```python
from build123d import *

# Parameters (mm, degrees)
SKETCH1_W               = 57.15
SKETCH1_H               = 18.542
BOSS_EXTRUDE1_DEPTH     = 19.05
CUT_EXTRUDE1_DEPTH      = 41.848617676
CUT_EXTRUDE1_DEPTH_BACK = 41.848617676
CUT_EXTRUDE2_DEPTH      = 4.572
CUT_EXTRUDE2_DEPTH_BACK = 4.572
CUT_EXTRUDE3_DEPTH      = 3.81
CUT_EXTRUDE3_DEPTH_BACK = 3.81
CUT_EXTRUDE5_DEPTH      = 44.89150133
FILLET1_R               = 3.175
SKETCH9_R               = 3.96875
CUT_EXTRUDE6_DEPTH      = 1.5875
SKETCH10_W              = 22.225
SKETCH10_H              = 6.096
CUT_EXTRUDE7_DEPTH      = 41.503184716
FILLET2_R               = 3.175
FILLET3_R               = 0.79375


with BuildPart() as part:
    # Sketch1 → Boss-Extrude1 (new body)
    with BuildSketch(Plane.XY):
        with Locations((6.35, 0)):
            Rectangle(SKETCH1_W, SKETCH1_H)
    extrude(amount=BOSS_EXTRUDE1_DEPTH)

    # Sketch3 → Cut-Extrude1 (cut, two sides: drawn at the far end of the back side and taken through both)
    with BuildSketch(Plane(origin=(0, 0, 0), x_dir=(1, 0, 0), z_dir=(0, 1, 0)).offset(-CUT_EXTRUDE1_DEPTH_BACK)):
        with BuildLine():
            Line((-5.1435, -19.05), (-5.1435, -14.2875))
            ThreePointArc((-5.1435, -14.2875), (0, -9.144), (5.1435, -14.2875))
            Line((5.1435, -14.2875), (5.1435, -19.05))
            ThreePointArc((5.1435, -19.05), (0, -24.1935), (-5.1435, -19.05))
        make_face()
    extrude(amount=CUT_EXTRUDE1_DEPTH + CUT_EXTRUDE1_DEPTH_BACK, mode=Mode.SUBTRACT)

    # Sketch5 → Cut-Extrude2 (cut, two sides: drawn at the far end of the back side and taken through both)
    with BuildSketch(Plane(origin=(0, 0, 0), x_dir=(1, 0, 0), z_dir=(0, 1, 0)).offset(-CUT_EXTRUDE2_DEPTH_BACK)):
        with BuildLine():
            Line((12.954, -14.2875), (12.954, -19.05))
            ThreePointArc((12.954, -19.05), (0, -32.004), (-12.954, -19.05))
            Line((-12.954, -19.05), (-12.954, -14.2875))
            ThreePointArc((-12.954, -14.2875), (0, -1.3335), (12.954, -14.2875))
        make_face()
        with BuildLine():
            Line((-6.731, -19.05), (-6.731, -14.2875))
            ThreePointArc((-6.731, -14.2875), (0, -7.5565), (6.731, -14.2875))
            Line((6.731, -14.2875), (6.731, -19.05))
            ThreePointArc((6.731, -19.05), (0, -25.781), (-6.731, -19.05))
        make_face(mode=Mode.SUBTRACT)
    extrude(amount=CUT_EXTRUDE2_DEPTH + CUT_EXTRUDE2_DEPTH_BACK, mode=Mode.SUBTRACT)

    # Sketch6 → Cut-Extrude3 (cut, two sides: drawn at the far end of the back side and taken through both)
    with BuildSketch(Plane(origin=(0, 0, 0), x_dir=(1, 0, 0), z_dir=(0, 1, 0)).offset(-CUT_EXTRUDE3_DEPTH_BACK)):
        with BuildLine():
            Line((-8.3185, -19.05), (-8.3185, -14.2875))
            ThreePointArc((-8.3185, -14.2875), (0, -5.969), (8.3185, -14.2875))
            Line((8.3185, -14.2875), (8.3185, -19.05))
            ThreePointArc((8.3185, -19.05), (0, -27.3685), (-8.3185, -19.05))
        make_face()
    extrude(amount=CUT_EXTRUDE3_DEPTH + CUT_EXTRUDE3_DEPTH_BACK, mode=Mode.SUBTRACT)

    # Sketch8 → Cut-Extrude5 (cut, through all)
    with BuildSketch(Plane.XZ.offset(9.271)):
        Polygon((-22.225, 19.05), (34.925, 19.05), (34.925, 6.803571429), align=None)
    extrude(amount=-CUT_EXTRUDE5_DEPTH, mode=Mode.SUBTRACT)

    # Fillet1
    fillet1_edges = [part.edges().sort_by_distance(p)[0] for p in [
        (-22.225, 0, 19.05),
        (34.925, 0, 6.803571429),
        (-22.225, 0, 0),
        (34.925, 0, 0),
    ]]
    fillet(fillet1_edges, radius=FILLET1_R)

    # Sketch9 → Cut-Extrude6 (cut)
    with BuildSketch(Plane(origin=(0, 0, 0), x_dir=(-1, 0, 0), z_dir=(0, 0, -1))):
        with Locations((-23.8125, 0)):
            Circle(SKETCH9_R)
    extrude(amount=-CUT_EXTRUDE6_DEPTH, mode=Mode.SUBTRACT)

    # Sketch10 → Cut-Extrude7 (cut, through all)
    with BuildSketch(Plane(origin=(0, 0, 0), x_dir=(-1, 0, 0), z_dir=(0, 0, -1))):
        with Locations((-23.8125, 6.223)):
            Rectangle(SKETCH10_W, SKETCH10_H)
        with Locations((-23.8125, -6.223)):
            Rectangle(SKETCH10_W, SKETCH10_H)
    extrude(amount=-CUT_EXTRUDE7_DEPTH, mode=Mode.SUBTRACT)

    # Fillet2
    fillet2_edges = [part.edges().sort_by_distance(p)[0] for p in [
        (12.7, 3.175, 5.783035714),
        (12.7, -3.175, 5.783035714),
    ]]
    fillet(fillet2_edges, radius=FILLET2_R)

    # Fillet3
    # the kernel refuses this fillet: 0.79375 mm, written as the material it adds along each edge
    with BuildSketch(Plane(origin=(-6.731, 4.572, 17.714232143), x_dir=(-1, 0, 0), z_dir=(0, 0, -1))) as fillet3_piece_1_section:
        with BuildLine():
            CenterArc((FILLET3_R, -FILLET3_R), FILLET3_R, 90, 90)
            Line((0, -FILLET3_R), (0, 0))
            Line((0, 0), (FILLET3_R, 0))
        make_face()
    fillet3_piece_1 = extrude(amount=3.426732143, mode=Mode.PRIVATE)
    fillet3_piece_1 = split(fillet3_piece_1, bisect_by=Plane(origin=(-6.763728877, 4.396665284, 15.736870474), z_dir=(-0.2095290887308735, 0, -0.9778024140774095)), keep=Keep.TOP, mode=Mode.PRIVATE)
    fillet3_piece_1 = split(fillet3_piece_1, bisect_by=Plane(origin=(-6.915533266, 3.81, 15.028449993), z_dir=(0, 1, 0)), keep=Keep.TOP, mode=Mode.PRIVATE)
    add(fillet3_piece_1)
    with BuildSketch(Plane(origin=(-6.731, -4.572, 17.714232143), x_dir=(-1, 0, 0), z_dir=(0, 0, -1))) as fillet3_piece_2_section:
        with BuildLine():
            CenterArc((FILLET3_R, FILLET3_R), FILLET3_R, 180, 90)
            Line((0, FILLET3_R), (0, 0))
            Line((0, 0), (FILLET3_R, 0))
        make_face()
    fillet3_piece_2 = extrude(amount=3.426732143, mode=Mode.PRIVATE)
    fillet3_piece_2 = split(fillet3_piece_2, bisect_by=Plane(origin=(-6.763728877, -4.396665284, 15.736870474), z_dir=(-0.2095290887308735, 0, -0.9778024140774095)), keep=Keep.TOP, mode=Mode.PRIVATE)
    fillet3_piece_2 = split(fillet3_piece_2, bisect_by=Plane(origin=(-6.915533266, -3.81, 15.028449993), z_dir=(0, -1, 0)), keep=Keep.TOP, mode=Mode.PRIVATE)
    add(fillet3_piece_2)
    with BuildSketch(Plane(origin=(-12.954, -4.572, 19.047732143), x_dir=(1, 0, 0), z_dir=(0, 0, -1))) as fillet3_piece_3_section:
        with BuildLine():
            CenterArc((FILLET3_R, -FILLET3_R), FILLET3_R, 90, 90)
            Line((0, -FILLET3_R), (0, 0))
            Line((0, 0), (FILLET3_R, 0))
        make_face()
    fillet3_piece_3 = extrude(amount=4.760232143, mode=Mode.PRIVATE)
    fillet3_piece_3 = split(fillet3_piece_3, bisect_by=Plane(origin=(-12.496129388, -4.39094469, 16.965242012), z_dir=(-0.2095290887308735, 0, -0.9778024140774095)), keep=Keep.TOP, mode=Mode.PRIVATE)
    add(fillet3_piece_3)
    with BuildSketch(Plane(origin=(-12.954, 4.572, 19.047732143), x_dir=(1, 0, 0), z_dir=(0, 0, -1))) as fillet3_piece_4_section:
        with BuildLine():
            CenterArc((FILLET3_R, FILLET3_R), FILLET3_R, 180, 90)
            Line((0, FILLET3_R), (0, 0))
            Line((0, 0), (FILLET3_R, 0))
        make_face()
    fillet3_piece_4 = extrude(amount=4.760232143, mode=Mode.PRIVATE)
    fillet3_piece_4 = split(fillet3_piece_4, bisect_by=Plane(origin=(-12.496129388, 4.39094469, 16.965242012), z_dir=(-0.2095290887308735, 0, -0.9778024140774095)), keep=Keep.TOP, mode=Mode.PRIVATE)
    add(fillet3_piece_4)
    with BuildSketch(Plane(origin=(0, 4.572, 14.2875), x_dir=(-1, 0, 0), z_dir=(0, 0, 1))) as fillet3_piece_5_section:
        with BuildLine():
            CenterArc((6.731 + FILLET3_R, FILLET3_R), FILLET3_R, 180, 90)
            Line((6.731 + FILLET3_R, 0), (6.731, 0))
            Line((6.731, 0), (6.731, FILLET3_R))
        make_face()
    fillet3_piece_5 = revolve(axis=Axis((0, 4.572, 14.2875), (0, -1, 0)), revolution_arc=167.905242923, mode=Mode.PRIVATE)
    fillet3_piece_5 = split(fillet3_piece_5, bisect_by=Plane(origin=(-0.733722895, 3.81, 7.361688783), z_dir=(0, 1, 0)), keep=Keep.TOP, mode=Mode.PRIVATE)
    add(fillet3_piece_5)
    with BuildSketch(Plane(origin=(0, -4.572, 14.2875), x_dir=(-1, 0, 0), z_dir=(0, 0, 1))) as fillet3_piece_6_section:
        with BuildLine():
            CenterArc((6.731 + FILLET3_R, -FILLET3_R), FILLET3_R, 90, 90)
            Line((6.731, -FILLET3_R), (6.731, 0))
            Line((6.731, 0), (6.731 + FILLET3_R, 0))
        make_face()
    fillet3_piece_6 = revolve(axis=Axis((0, -4.572, 14.2875), (0, -1, 0)), revolution_arc=167.905242923, mode=Mode.PRIVATE)
    fillet3_piece_6 = split(fillet3_piece_6, bisect_by=Plane(origin=(-0.733722895, -3.81, 7.361688783), z_dir=(0, -1, 0)), keep=Keep.TOP, mode=Mode.PRIVATE)
    add(fillet3_piece_6)
    with BuildSketch(Plane(origin=(0, -4.572, 14.2875), x_dir=(-1, 0, 0), z_dir=(0, 0, 1))) as fillet3_piece_7:
        with BuildLine():
            CenterArc((12.954 - FILLET3_R, -FILLET3_R), FILLET3_R, 0, 90)
            Line((12.954 - FILLET3_R, 0), (12.954, 0))
            Line((12.954, 0), (12.954, -FILLET3_R))
        make_face()
    revolve(axis=Axis((0, -4.572, 14.2875), (0, -1, 0)), revolution_arc=167.905242923)
    with BuildSketch(Plane(origin=(0, 4.572, 14.2875), x_dir=(-1, 0, 0), z_dir=(0, 0, 1))) as fillet3_piece_8:
        with BuildLine():
            CenterArc((12.954 - FILLET3_R, FILLET3_R), FILLET3_R, 270, 90)
            Line((12.954, FILLET3_R), (12.954, 0))
            Line((12.954, 0), (12.954 - FILLET3_R, 0))
        make_face()
    revolve(axis=Axis((0, 4.572, 14.2875), (0, -1, 0)), revolution_arc=167.905242923)


solid = part.part
```
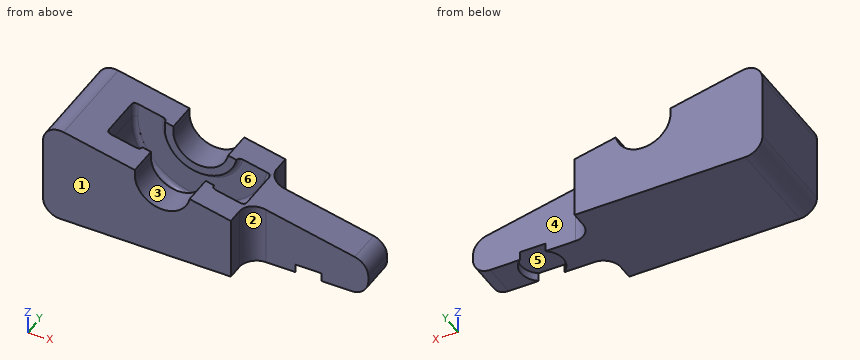
CAD build for the part. Positions are in the model's coordinates, mm. Face numbers are marked on the shaded views. A direction names the side the tool comes from. Round coordinates to 2 decimals unless told otherwise and drop trailing zeros. Loops run counter-clockwise (first coordinate to the right, second up) from the corner with the lowest first, then second, coordinate; pieces in that order, holes last. Notation, with made-up numbers: M -19.5,-3.75 L 30.5,-3.75 A28 cw 30.5,22.25 Z; hole C -31,-35 d5. An arc over 180 degrees is marked long. Return JSON: item names as keys, results as strings. Group by question number.
(1) Mould opens along X. For the marked faces 1, 2 and 3 say: +X half, -X half, draft (parallel to the pull), parting line (faces both ways), or undercut.
(2) Wall check: probe 1 along Y at (x, z) = (5.5, 5); probe 2 along Y at (x, z) = (26.5, 6.5) (3 decimals); probe 3 along X at (y, z) = (-7.5, 10) (3 decimals). Give the ranges that are in metal, low to high. Write a range as [from, to].
(3) Drop flat-ended pins along their axis: P1, Ø1.2, axis at y = -5.5, z = 14.5, coming from the +X side; P2, Ø8.5, axis at x = 22.5, z = 4.5, coming from the +Y side (3 decimals); P3, Ø2, axis at y = -6, z = 5, coming from the +X side. Give the stop position or say it passes through.
(4) Saw through at D-D, the plane x = -13.5. List the corners of the cut face in (y, z), and give its area (3 significant figures).
(5) Saw through at B-B, the plane x = 17.5. List the corners of the cut face in (y, z) (1 decimal), and give its area (3 significant figures).
(6) Tool access for the marked faces 4, 5 and 6: list every direction of +Z, -Z, +X, -X, +Y, -Y with a clear straight run to the whole face (end or side of a thin tool).
Answer list:
{
 "1": {"face 1": "draft", "face 2": "+X half", "face 3": "undercut"},
 "2": {"probe 1": "[-9.27, -4.57], [4.57, 9.27]", "probe 2": "[-3.175, 3.175]", "probe 3": "[-22.225, -2.841], [2.841, 12.7]"},
 "3": {"P1": "x = -5.13", "P2": "y = 3.175", "P3": "x = 13"},
 "4": {"outline": "M -9.27,0 L 9.27,0 L 9.27,17.18 L -9.27,17.18 Z", "area": "319 mm2"},
 "5": {"outline": "M -3.2,0 L 3.2,0 L 3.2,10.5 L -3.2,10.5 Z", "area": "66.9 mm2"},
 "6": {"face 4": "+Z, -Z, +X, +Y", "face 5": "-Z", "face 6": "none"}
}
